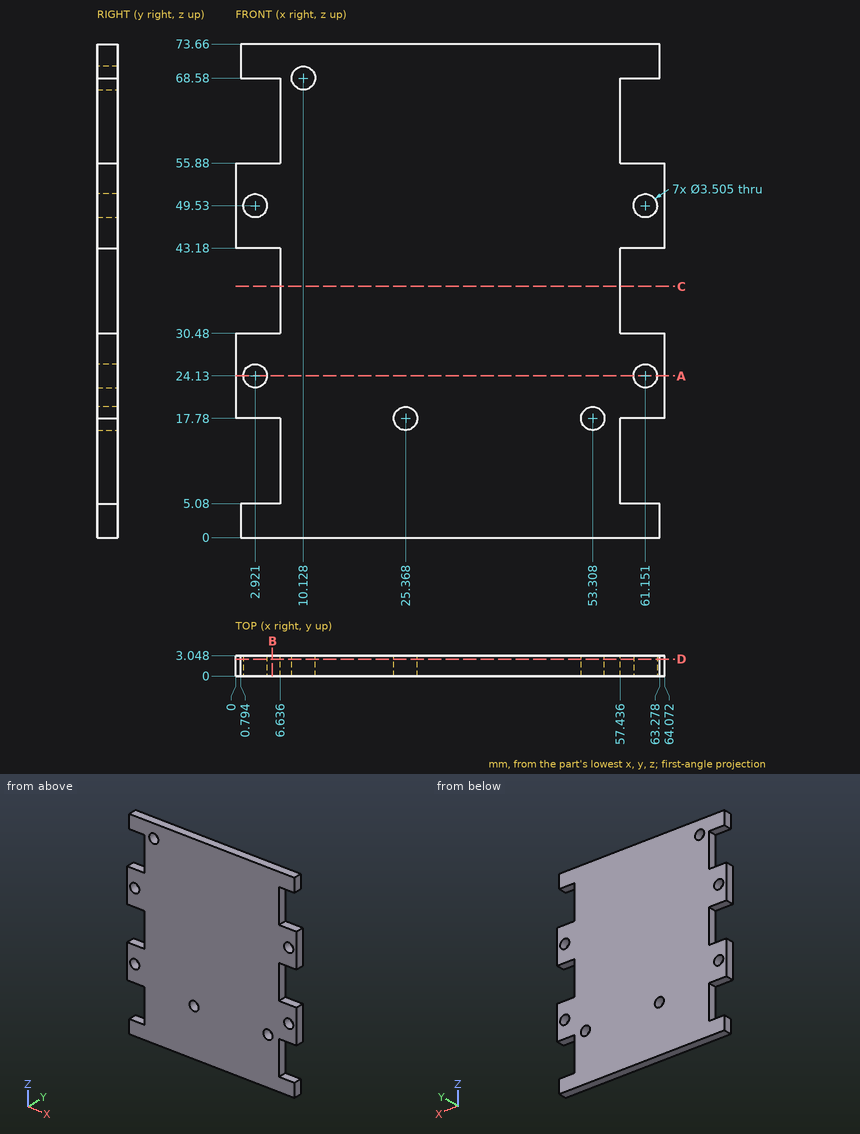
For this review, use the dimensioned drawing (mm, ordinates from the lowest corner) and the shaded views. Round coordinates to 2 decimals unless told otherwise and drop trailing zeros. Write each loop counter-clockwise with the first axis right and the second up, starting at its lowest first coordinate (ties: lowest second). Pieces come first, ordered by that corner, then holes. Notation, with made-up numbers: (21, 0.5) -> (44, 0.5) arc R28 ccw to (44, 23.5) -> close; hole circle Ø9 at (1, 69.5). An arc over 180 degrees is marked (long way). Use CSV: the item, a comma, the result in double quotes.
Q1. Consider section B-B (x = 5.5). Give the boundary of the cut face in (y, z), then the cut area to 3 significant figures.
Checks:
outline,"(0, 0) -> (3.05, 0) -> (3.05, 5.08) -> (0, 5.08) -> close; (0, 17.78) -> (3.05, 17.78) -> (3.05, 30.48) -> (0, 30.48) -> close; (0, 43.18) -> (3.05, 43.18) -> (3.05, 55.88) -> (0, 55.88) -> close; (0, 68.58) -> (3.05, 68.58) -> (3.05, 73.66) -> (0, 73.66) -> close"
area,"108 mm²"
Q2. To check wall thickness, follow probe 1 along Z at (x, y) = (58.5, 0.95); probe 2 along X at (y, z) = (0.9, 24.13); probe 3 along Z at (x, y) = (53.5, 1.75). State the ranges of each line that lie inside material, in increasing order. Write a range as [from, to].
Checks:
probe 1,"[0, 5.08], [17.78, 30.48], [43.18, 55.88], [68.58, 73.66]"
probe 2,"[0, 1.17], [4.67, 59.4], [62.9, 64.07]"
probe 3,"[0, 16.04], [19.52, 73.66]"
Q3. For pin 1 Ø0.9 at (y, z) = (1, 3) entering from -X; pin 2 Ø0.9 at (y, z) = (2, 2.5) entering from +X; pin 3 Ø3 at (x, z) = (61.15, 49.53) entering from +Y; pin 4 Ø1.5 at (y, z) = (2, 9) entering from -X, all flat-tipped, find the tip position at first contact; note any pin that passes through.
Checks:
pin 1,"x = 0.79"
pin 2,"x = 63.28"
pin 3,"through"
pin 4,"x = 6.64"
Q4. Consider section C-C (z = 37.5). Give the boundary of the cut face in (x, y) (1 decimal), then the cut area to 3 significant figures.
Checks:
outline,"(6.6, 0) -> (57.4, 0) -> (57.4, 3) -> (6.6, 3) -> close"
area,"155 mm²"
Q5. Consider section A-A (z = 24.13). Give the boundary of the cut face in (x, y).
Checks:
outline,"(0, 0) -> (1.17, 0) -> (1.17, 3.05) -> (0, 3.05) -> close; (4.67, 0) -> (59.4, 0) -> (59.4, 3.05) -> (4.67, 3.05) -> close; (62.9, 0) -> (64.07, 0) -> (64.07, 3.05) -> (62.9, 3.05) -> close"
Q6. Consider section D-D (y = 2.5). State how many separate pieces and enclosed holes the cut face has, then the cut area to 3 significant figures.
Checks:
separate pieces,"1"
enclosed holes,"7"
area,"4,130 mm²"
